from build123d import *

# Parameters (mm, degrees)
BOSS_EXTRUDE1_DEPTH     = 88.9
CUT_EXTRUDE1_DEPTH      = 3.048
CUT_EXTRUDE1_DEPTH_BACK = 36.576
SKETCH3_W               = 76.2
SKETCH3_H               = 94.842471145


with BuildPart() as part:
    # Sketch1 → Boss-Extrude1 (new body)
    with BuildSketch(Plane.XY):
        with BuildLine():
            ThreePointArc((25.4, 0), (17.960512242, -17.960512242), (0, -25.4))
            Line((0, -25.4), (69.126967967, -107.78231242))
            Line((69.126967967, -107.78231242), (101.091555285, -80.96083899))
            Line((101.091555285, -80.96083899), (19.457528855, 16.326805286))
            ThreePointArc((19.457528855, 16.326805286), (23.868192568, 8.68731164), (25.4, 0))
        make_face()
        with BuildLine():
            ThreePointArc((19.457528855, 16.326805286), (0, 25.4), (-19.457528855, 16.326805286))
            Line((-19.457528855, 16.326805286), (0, 0))
            Line((0, 0), (19.457528855, 16.326805286))
        make_face()
        with BuildLine():
            Line((12.507058463, -10.494668144), (0, -25.4))
            ThreePointArc((0, -25.4), (17.960512242, -17.960512242), (25.4, 0))
            ThreePointArc((25.4, 0), (23.868192568, 8.68731164), (19.457528855, 16.326805286))
            Line((19.457528855, 16.326805286), (0, 0))
            Line((0, 0), (12.507058463, -10.494668144))
        make_face()
        Polygon((-12.507058463, -10.494668144), (0, -25.4), (12.507058463, -10.494668144), (0, 0), align=None)
        with BuildLine():
            ThreePointArc((-19.457528855, 16.326805286), (-23.020217791, -10.734503848), (0, -25.4))
            Line((0, -25.4), (-12.507058463, -10.494668144))
            Line((-12.507058463, -10.494668144), (0, 0))
            Line((0, 0), (-19.457528855, 16.326805286))
        make_face()
        with BuildLine():
            Line((-69.126967967, -107.78231242), (0, -25.4))
            ThreePointArc((0, -25.4), (-23.020217791, -10.734503848), (-19.457528855, 16.326805286))
            Line((-19.457528855, 16.326805286), (-101.091555285, -80.96083899))
            Line((-101.091555285, -80.96083899), (-69.126967967, -107.78231242))
        make_face()
    extrude(amount=BOSS_EXTRUDE1_DEPTH)

    # Sketch3 → Cut-Extrude1 (cut, two sides: drawn at the far end of the back side and taken through both)
    with BuildSketch(Plane(origin=(12.507058463, -10.494668144, 0), x_dir=(0, 0, -1), z_dir=(0.7660444431189793, -0.6427876096865378, 0)).offset(-CUT_EXTRUDE1_DEPTH_BACK)):
        with Locations((-44.45, -73.228764428)):
            Rectangle(SKETCH3_W, SKETCH3_H)
    extrude(amount=CUT_EXTRUDE1_DEPTH + CUT_EXTRUDE1_DEPTH_BACK, mode=Mode.SUBTRACT)


solid = part.part
Geometry check sheet. Reference: the model listing, model coordinates, mm. A direction names the side the tool comes from. Give positions to 0.01 mm unless a question says otherwise; leave off trailing zeros. Order: outer loops, then holes, each group sorted by start corner. A loop starts at its lowest first (then second) coordinate and runs counter-clockwise, first axis right, second up.
1. Depth check by flat-ended pin: pin 1 (8 mm diameter, centred on y = -87.5, z = 77, fed in from +X); pin 2 (4 mm diameter, centred on x = -62, z = 17.5, fed in from +Y); pin 3 (5 mm diameter, centred on x = 1, z = 24.5, fed in from -Y); pin 4 (10 mm diameter, centred on x = 54, y = -86.5, fed in from -Z). Enter the tip coordinate at first touch or a pass-through.
Completed:
pin 1: stops at x = 98.07
pin 2: stops at y = -31.99
pin 3: stops at y = -29.57
pin 4: stops at z = 0
2. Draft check along Z on faces 1 (the face through (-1, -25, 88.9)), 2 (the face through (34.08, -66.014, 43.828)), 3 (the face through (-62.156, -42.572, 44.983)). Enter one of: pulls with the +Z half, pulls with the -Z half, needs draft (parallel to the pull), parting line crosses it, or undercut.
Completed:
face 1: pulls with the +Z half
face 2: needs draft
face 3: undercut
3. Access from +Z, -Z, +X, -X, +Y, -Y to the whole of each face (thin tool, end or side, straight path). Record for faces 4 (the face through (-49, -55, 82.55)), 5 (the face through (0.3, 25.4, 43.8)), 6 (the face through (-1, -25, 0)), 7 (the face through (-34.72, -66.78, 4.73)), 8 (the face through (-18.29, -18.34, 44.98)).
Completed:
face 4: none
face 5: +Z, -Z, +Y
face 6: -Z, +X, -X, +Y, -Y
face 7: +Z, -Z, -Y
face 8: -Y
4. Sectioned sample at D-D (x = 86). Record the boundary of the cut face in (y, z), then the cut area to 3 significant figures.
Completed:
outline: (-93.62, 0) - (-62.98, 0) - (-62.98, 88.9) - (-93.62, 88.9) - close
area: 2,720 mm2
5. Sectioned sample at A-A (z = 23.5). Record the boundary of the cut face in (x, y).
Completed:
outline: (-101.09, -80.96) - (-69.13, -107.78) - (-65.05, -102.92) - (-93.06, -79.41) - (-32.1, -6.75) - (-4.08, -30.26) - (0, -25.4) - (69.13, -107.78) - (101.09, -80.96) - (19.46, 16.33) arc R25.4 ccw to (-19.46, 16.33) - close
6. Sectioned sample at B-B (y = -11.5). Record the boundary of the cut face in (x, z).
Completed:
outline: (-42.81, 0) - (42.81, 0) - (42.81, 88.9) - (-42.81, 88.9) - close; hole (-36.08, 6.35) - (-26.44, 6.35) - (-26.44, 82.55) - (-36.08, 82.55) - close
7. Scan lines: line 1 (Z direction, x = -38.5, y = -38.5); line 2 (X direction, y = -29, z = 30.5); line 3 (X direction, y = -9, z = 36.5). Record each from-to range of solid material in increasing order.
Completed:
line 1: z = 0 to 6.35, 82.55 to 88.9
line 2: x = -57.49 to -50.77, -5.59 to -3.02, 3.02 to 57.49
line 3: x = -40.71 to -33.99, -29.42 to 40.71
8. Sectioned sample at C-C (y = -54). Record the boundary of the cut face in (x, z).
Completed:
outline: (-78.47, 0) - (-24, 0) - (-24, 6.35) - (-71.74, 6.35) - (-71.74, 82.55) - (-24, 82.55) - (-24, 88.9) - (-78.47, 88.9) - close; (24, 0) - (78.47, 0) - (78.47, 88.9) - (24, 88.9) - close
